CAD build for the part. Positions are in the model's coordinates, mm. Coordinates: 2 decimals unless noted, no trailing zeros. Write each loop counter-clockwise with the first axis right and the second up, starting at its lowest first coordinate (ties: lowest second). Pieces come first, ordered by that corner, then holes. Notation, with made-up numbers: (-6, -18) - (4, -18) arc R25 cw to (4, 12) - close; hole circle Ø5 at (67.25, 29.5). An arc over 180 degrees is marked (long way). Answer in a Markdown table with one row per item. Add a question column.
Q1. Band-saw the part on B-B (z = 6). State how many separate pieces and enclosed holes the cut face has, and give its area (3 significant figures).
Q2. Pin check, flat tip, straight feed: pin 1 (4.5 mm diameter, centred on x = 11, y = 16, fed in from +Z). Stop position of the tip, or through.
Q3. Drill centre lines: line 1 along X through (y, z) = (-19, 0.5); line 2 along X through (y, z) = (-45, 1.25); line 3 along X through (y, z) = (-41.5, 2). Where is each one in solid material? Low to high. Write a range as from..to.
Q4. Band-saw the part on A-A (y = -20). List the corners of the cut face in (x, z), and give its area (3 significant figures).
```python
from build123d import *

# Parameters (mm, degrees)
SKETCH1_W           = 65
SKETCH1_H           = 460
SKETCH1_R           = 2.54
SKETCH1_R_2         = 6
SKETCH1_R_3         = 2
SKETCH1_R_4         = 12.7
BOSS_EXTRUDE1_DEPTH = 10


with BuildPart() as part:
    # Sketch1 → Boss-Extrude1 (new body)
    with BuildSketch(Plane.XY):
        with Locations((0, -191.425)):
            Rectangle(SKETCH1_W, SKETCH1_H)
        with Locations((-23.5712, 3.5712)):
            Circle(SKETCH1_R, mode=Mode.SUBTRACT)
        with Locations((23.5712, 3.5712)):
            Circle(SKETCH1_R, mode=Mode.SUBTRACT)
        with Locations((23.5712, -43.5712)):
            Circle(SKETCH1_R, mode=Mode.SUBTRACT)
        with Locations((-23.5712, -43.5712)):
            Circle(SKETCH1_R, mode=Mode.SUBTRACT)
        with Locations((0, -106)):
            Circle(SKETCH1_R_2, mode=Mode.SUBTRACT)
        with Locations((11, -106)):
            Circle(SKETCH1_R_3, mode=Mode.SUBTRACT)
        with Locations((0, -20)):
            Circle(SKETCH1_R_4, mode=Mode.SUBTRACT)
        with Locations((0, -95)):
            Circle(SKETCH1_R_3, mode=Mode.SUBTRACT)
        with Locations((0, 16)):
            Circle(SKETCH1_R_2, mode=Mode.SUBTRACT)
        with Locations((11, 16)):
            Circle(SKETCH1_R_3, mode=Mode.SUBTRACT)
        with Locations((-11, -106)):
            Circle(SKETCH1_R_3, mode=Mode.SUBTRACT)
        with Locations((0, 27)):
            Circle(SKETCH1_R_3, mode=Mode.SUBTRACT)
        with Locations((-11, 16)):
            Circle(SKETCH1_R_3, mode=Mode.SUBTRACT)
    extrude(amount=BOSS_EXTRUDE1_DEPTH)


solid = part.part
```
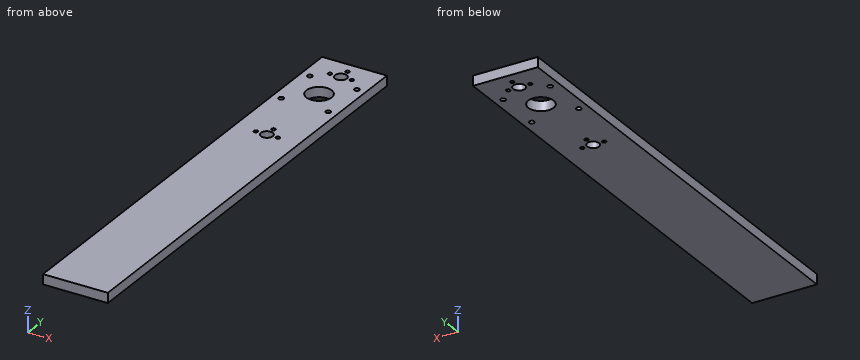
Checked values:
| question | item | result |
|---|---|---|
| 1 | separate pieces | 1 |
| 1 | enclosed holes | 13 |
| 1 | area | 29,000 mm² |
| 2 | pin 1 | stops at z = 10 |
| 3 | line 1 | x = -32.5..-12.66, 12.66..32.5 |
| 3 | line 2 | x = -32.5..-25.67, -21.47..21.47, 25.67..32.5 |
| 3 | line 3 | x = -32.5..-25.04, -22.1..22.1, 25.04..32.5 |
| 4 | outline | (-32.5, 0) - (-12.7, 0) - (-12.7, 10) - (-32.5, 10) - close; (12.7, 0) - (32.5, 0) - (32.5, 10) - (12.7, 10) - close |
| 4 | area | 396 mm² |
